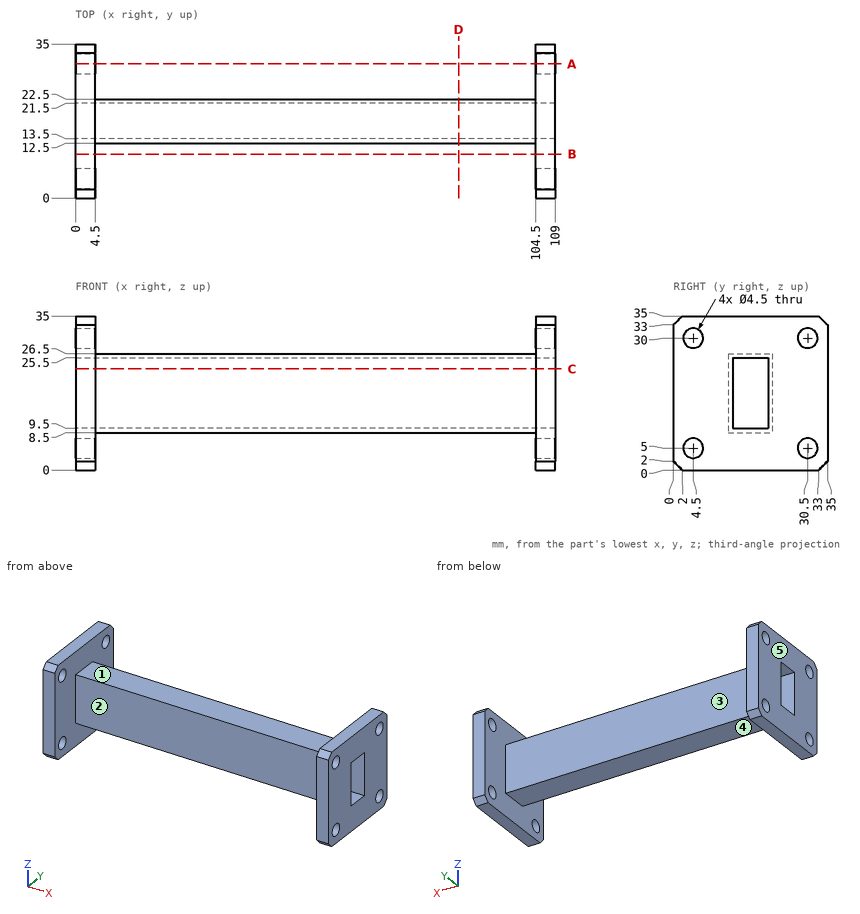
The drawing under review shows one solid part. Ordinate dimensions are in mm from its lowest x, y, z. A direction names the side the tool comes from. Give positions to 0.01 mm unless a question says otherwise; leave off trailing zeros. Loops run counter-clockwise (first coordinate to the right, second up) from the corner with the lowest first, then second, coordinate; pieces in that order, holes last. Notation, with made-up numbers: M 28,1.5 L 35,1.5 A18 cw 35,15.5 Z; hole C -33,-27.5 d4. An arc over 180 degrees is marked long. One line per item, written item: value. Start each with the question number.
Q1. Add section B-B (y = 10). Give the boundary of the cut face in (x, z), and give its area (3 significant figures).
Q2. Machinability: for the marked faces 1, 2, 3, 4 and 5, which of the approach directions +Z, -Z, +X, -X, +Y, -Y give a long, thin tool a straight path to every point of the face, cutting with its end or side? Answer none if there is none.
Q3. For L1, parallel to Z at x = 107.85, y = 4.5; L2, parallel to Y at x = 107, z = 30; L3, parallel to X at y = 6, z = 18, list the stretches that pass through material, from the lowest coordinate up.
Q4. Add section A-A (y = 30.5). Give the boundary of the cut face in (x, z), and give its area (3 significant figures).
Q5. Clearance check with flat-ended pins moving along their axes: pin 1 Ø5.5 at (x, z) = (31.5, 19.5) entering from -Y; pin 2 Ø17.5 at (x, z) = (31.5, 21) entering from +Y; pin 3 Ø9 at (x, y) = (51.5, 17) entering from -Z; pin 4 Ø3.5 at (y, z) = (30.5, 30) entering from +X. State where each tip first meets the part, or that it passes through.
Q6. Add section D-D (x = 87). Give the boundary of the cut face in (y, z), and give its area (3 significant figures).
Q7. Add section C-C (z = 23). Give the boundary of the cut face in (x, y), and give its area (3 significant figures).
Reply:
1. outline: M 0,0 L 4.5,0 L 4.5,35 L 0,35 Z; M 104.5,0 L 109,0 L 109,35 L 104.5,35 Z
1. area: 315 mm²
2. face 1: +Z, +Y, -Y
2. face 2: +Z, -Z, -Y
2. face 3: +Z, -Z, +Y
2. face 4: -Z, +Y, -Y
2. face 5: +Z, -Z, -X, +Y, -Y
3. L1: 0 to 2.75, 7.25 to 27.75, 32.25 to 35
3. L2: 0 to 2.25, 6.75 to 28.25, 32.75 to 35
3. L3: 0 to 4.5, 104.5 to 109
4. outline: M 0,0 L 4.5,0 L 4.5,2.75 L 0,2.75 Z; M 0,7.25 L 4.5,7.25 L 4.5,27.75 L 0,27.75 Z; M 0,32.25 L 4.5,32.25 L 4.5,35 L 0,35 Z; M 104.5,0 L 109,0 L 109,2.75 L 104.5,2.75 Z; M 104.5,7.25 L 109,7.25 L 109,27.75 L 104.5,27.75 Z; M 104.5,32.25 L 109,32.25 L 109,35 L 104.5,35 Z
4. area: 234 mm²
5. pin 1: y = 12.5
5. pin 2: y = 22.5
5. pin 3: z = 8.5
5. pin 4: through
6. outline: M 12.5,8.5 L 22.5,8.5 L 22.5,26.5 L 12.5,26.5 Z; hole M 13.5,9.5 L 21.5,9.5 L 21.5,25.5 L 13.5,25.5 Z
6. area: 52.0 mm²
7. outline: M 0,0 L 4.5,0 L 4.5,12.5 L 104.5,12.5 L 104.5,0 L 109,0 L 109,13.5 L 0,13.5 Z; M 0,21.5 L 109,21.5 L 109,35 L 104.5,35 L 104.5,22.5 L 4.5,22.5 L 4.5,35 L 0,35 Z
7. area: 443 mm²
